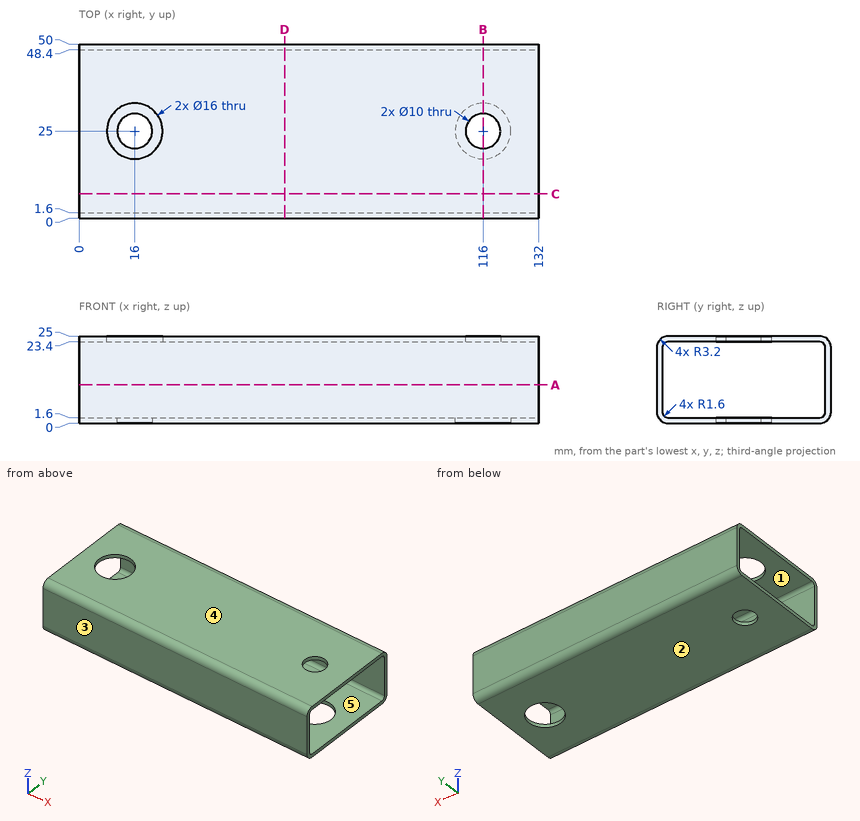
Source: three-view drawing plus pictorial views. Frame: mm from the lowest corner of the part. A direction names the side the tool comes from. Give positions to 0.01 mm unless a question says otherwise; leave off trailing zeros. Loops run counter-clockwise (first coordinate to the right, second up) from the corner with the lowest first, then second, coordinate; pieces in that order, holes last.
1) Line query: L1, parallel to Z at x = 126, y = 13; L2, parallel to Y at x = 79, z = 18; L3, parallel to Y at x = 16, z = 24.5. Output: solid intervals per line, ascending.
A:
L1: z = 0 to 1.6, 23.4 to 25
L2: y = 0 to 1.6, 48.4 to 50
L3: y = 1.48 to 17, 33 to 48.52
2) Section query B-B on x = 116. Return the cut outline in (y, z), and give its area (3 significant figures).
A:
outline: (0, 3.2) arc R3.2 ccw to (3.2, 0) - (17, 0) - (17, 1.6) - (3.2, 1.6) arc R1.6 cw to (1.6, 3.2) - (1.6, 21.8) arc R1.6 cw to (3.2, 23.4) - (20, 23.4) - (20, 25) - (3.2, 25) arc R3.2 ccw to (0, 21.8) - close; (30, 23.4) - (46.8, 23.4) arc R1.6 cw to (48.4, 21.8) - (48.4, 3.2) arc R1.6 cw to (46.8, 1.6) - (33, 1.6) - (33, 0) - (46.8, 0) arc R3.2 ccw to (50, 3.2) - (50, 21.8) arc R3.2 ccw to (46.8, 25) - (30, 25) - close
area: 182 mm2
3) Section query A-A on z = 11. Return the cut outline in (x, y), and give its area (3 significant figures).
A:
outline: (0, 0) - (132, 0) - (132, 1.6) - (0, 1.6) - close; (0, 48.4) - (132, 48.4) - (132, 50) - (0, 50) - close
area: 422 mm2
4) Contact query for flat-ended pins moving along their axis: pin 1 (14.5 mm diameter, centred on x = 116, y = 25, fed in from -Z); pin 2 (1 mm diameter, centred on y = 13.5, z = 3, fed in from -X). Output: stop coordinate, or through.
A:
pin 1: stops at z = 23.4
pin 2: passes through
5) Section query C-C on y = 7. Return the cut outline in (x, z).
A:
outline: (0, 0) - (132, 0) - (132, 1.6) - (0, 1.6) - close; (0, 23.4) - (132, 23.4) - (132, 25) - (0, 25) - close
6) Reachability of the marked faces 4 and 5 from +Z, -Z, +X, -X, +Y, -Y: full face, straight path, thin tool, end or side. Return the list, or none.
A:
face 4: +Z, +X, -X, +Y, -Y
face 5: +X, -X
7) Section query D-D on x = 59. Return the cut outline in (y, z).
A:
outline: (0, 3.2) arc R3.2 ccw to (3.2, 0) - (46.8, 0) arc R3.2 ccw to (50, 3.2) - (50, 21.8) arc R3.2 ccw to (46.8, 25) - (3.2, 25) arc R3.2 ccw to (0, 21.8) - close; hole (1.6, 3.2) arc R1.6 ccw to (3.2, 1.6) - (46.8, 1.6) arc R1.6 ccw to (48.4, 3.2) - (48.4, 21.8) arc R1.6 ccw to (46.8, 23.4) - (3.2, 23.4) arc R1.6 ccw to (1.6, 21.8) - close
8) Mould query, pull axis Y, two halves, no side actions, for the marked faces 1, 2 and 3. Classes: released by +Y, released by -Y, zero draft, split by the parting line, or undercut.
A:
face 1: undercut
face 2: zero draft
face 3: released by -Y
